```python
from build123d import *

# Parameters (mm, degrees)
BOSS_EXTRUDE1_DEPTH = 90
SKETCH2_R           = 4.5
CUT_EXTRUDE1_DEPTH  = 10
SKETCH3_R           = 4.5
CUT_EXTRUDE2_DEPTH  = 95


with BuildPart() as part:
    # Sketch1 → Boss-Extrude1 (new body)
    with BuildSketch(Plane(origin=(0, 0, 0), x_dir=(1, 0, 0), z_dir=(0, 1, 0))):
        with BuildLine():
            Line((-20.25, -31.75), (20.25, -31.75))
            ThreePointArc((20.25, -31.75), (24.846194078, -29.846194078), (26.75, -25.25))
            Line((26.75, -25.25), (26.75, 25.25))
            ThreePointArc((26.75, 25.25), (24.846194078, 29.846194078), (20.25, 31.75))
            Line((20.25, 31.75), (-20.25, 31.75))
            ThreePointArc((-20.25, 31.75), (-24.846194078, 29.846194078), (-26.75, 25.25))
            Line((-26.75, 25.25), (-26.75, -25.25))
            ThreePointArc((-26.75, -25.25), (-24.846194078, -29.846194078), (-20.25, -31.75))
        make_face()
        with BuildLine():
            Line((-20.25, -30.25), (20.25, -30.25))
            ThreePointArc((20.25, -30.25), (23.785533906, -28.785533906), (25.25, -25.25))
            Line((25.25, -25.25), (25.25, 25.25))
            ThreePointArc((25.25, 25.25), (23.785533906, 28.785533906), (20.25, 30.25))
            Line((20.25, 30.25), (-20.25, 30.25))
            ThreePointArc((-20.25, 30.25), (-23.785533906, 28.785533906), (-25.25, 25.25))
            Line((-25.25, 25.25), (-25.25, -25.25))
            ThreePointArc((-25.25, -25.25), (-23.785533906, -28.785533906), (-20.25, -30.25))
        make_face(mode=Mode.SUBTRACT)
    extrude(amount=BOSS_EXTRUDE1_DEPTH)

    # Sketch2 → Cut-Extrude1 (cut)
    with BuildSketch(Plane.ZY.offset(34.75)):
        with Locations((0, 70)):
            Circle(SKETCH2_R)
        with Locations((0, 20)):
            Circle(SKETCH2_R)
    extrude(amount=-CUT_EXTRUDE1_DEPTH, mode=Mode.SUBTRACT)

    # Sketch3 → Cut-Extrude2 (cut)
    with BuildSketch(Plane.XY.offset(32.25)):
        with Locations((-11.2, 80)):
            Circle(SKETCH3_R)
        with Locations((-11.2, 10)):
            Circle(SKETCH3_R)
        with Locations((-11.2, 45)):
            Circle(SKETCH3_R)
    extrude(amount=-CUT_EXTRUDE2_DEPTH, mode=Mode.SUBTRACT)


solid = part.part
```
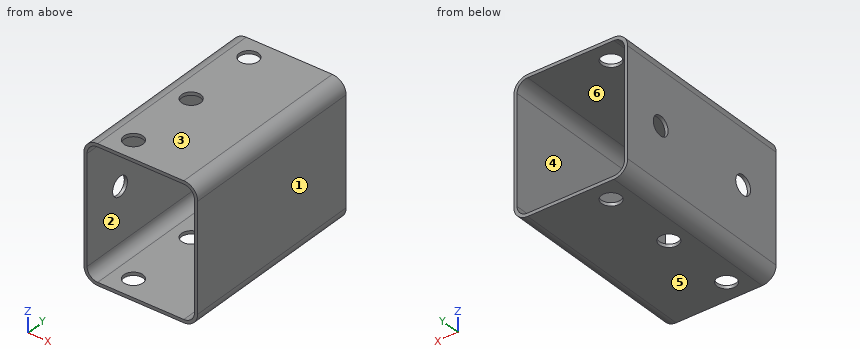
Check sheet for the modelled part. Datum: model origin and axes. Units: mm. Face numbers are marked on the shaded views. A direction names the side the tool comes from. Coordinates: 2 decimals unless noted, no trailing zeros. Write each loop counter-clockwise with the first axis right and the second up, starting at its lowest first coordinate (ties: lowest second). Pieces come first, ordered by that corner, then holes. Notation, with made-up numbers: (8, -13.75) -> (43, -13.75) arc R35 ccw to (43, 19.25) -> close; hole circle Ø2 at (81, 61). An arc over 180 degrees is marked (long way). Use a Markdown table: item, result.
1. Sectioned sample at D-D (x = -11.2). Give the number of separate pieces and of enclosed holes in the cut face, plus the area to 3 significant figures.
Reported:
| item | result |
|---|---|
| separate pieces | 8 |
| enclosed holes | 0 |
| area | 189 mm2 |
2. Sectioned sample at A-A (z = -15). Enter the section's corners in (x, y), plus the area to 3 significant figures.
Reported:
| item | result |
|---|---|
| outline | (-26.75, 0) -> (-25.25, 0) -> (-25.25, 90) -> (-26.75, 90) -> close; (25.25, 0) -> (26.75, 0) -> (26.75, 90) -> (25.25, 90) -> close |
| area | 270 mm2 |
3. Release check for a two-part mould opening along Z. For the marked faces 1, 2, 3 and 4 record: pulls with the +Z half, pulls with the -Z half, needs draft (parallel to the pull), parting line crosses it, or undercut.
Reported:
| item | result |
|---|---|
| face 1 | needs draft |
| face 2 | undercut |
| face 3 | pulls with the +Z half |
| face 4 | undercut |
4. Tool access check on the marked faces 5 and 6. Record the directions out of +Z, -Z, +X, -X, +Y, -Y that give a thin tool (end or side, any length) a straight path to the whole face; none if there is none.
Reported:
| item | result |
|---|---|
| face 5 | -Z, +X, -X, +Y, -Y |
| face 6 | +Y, -Y |
5. Sectioned sample at C-C (z = 0). Enter the section's corners in (x, y), plus the area to 3 significant figures.
Reported:
| item | result |
|---|---|
| outline | (-26.75, 0) -> (-25.25, 0) -> (-25.25, 15.5) -> (-26.75, 15.5) -> close; (-26.75, 24.5) -> (-25.25, 24.5) -> (-25.25, 65.5) -> (-26.75, 65.5) -> close; (-26.75, 74.5) -> (-25.25, 74.5) -> (-25.25, 90) -> (-26.75, 90) -> close; (25.25, 0) -> (26.75, 0) -> (26.75, 90) -> (25.25, 90) -> close |
| area | 243 mm2 |
6. Go/stop test with a flat-tipped pin: pin 1 Ø8 at (y, z) = (70, 0) entering from -X. Record where the tip stops, or that it passes through.
Reported:
| item | result |
|---|---|
| pin 1 | stops at x = 25.25 |
7. Sectioned sample at B-B (y = 10). Enter the section's corners in (x, z).
Reported:
| item | result |
|---|---|
| outline | (-26.75, -25.25) arc R6.5 ccw to (-20.25, -31.75) -> (-15.7, -31.75) -> (-15.7, -30.25) -> (-20.25, -30.25) arc R5 cw to (-25.25, -25.25) -> (-25.25, 25.25) arc R5 cw to (-20.25, 30.25) -> (-15.7, 30.25) -> (-15.7, 31.75) -> (-20.25, 31.75) arc R6.5 ccw to (-26.75, 25.25) -> close; (-6.7, -31.75) -> (20.25, -31.75) arc R6.5 ccw to (26.75, -25.25) -> (26.75, 25.25) arc R6.5 ccw to (20.25, 31.75) -> (-6.7, 31.75) -> (-6.7, 30.25) -> (20.25, 30.25) arc R5 cw to (25.25, 25.25) -> (25.25, -25.25) arc R5 cw to (20.25, -30.25) -> (-6.7, -30.25) -> close |
8. Scan lines: line 1 along Y through (x, z) = (-11.2, 31.3); line 2 along Z through (x, y) = (-7, 35.5); line 3 along X through (y, z) = (59, -10.5). Record each from-to range of solid material in increasing order.
Reported:
| item | result |
|---|---|
| line 1 | y = 0 to 5.5, 14.5 to 40.5, 49.5 to 75.5, 84.5 to 90 |
| line 2 | z = -31.75 to -30.25, 30.25 to 31.75 |
| line 3 | x = -26.75 to -25.25, 25.25 to 26.75 |
